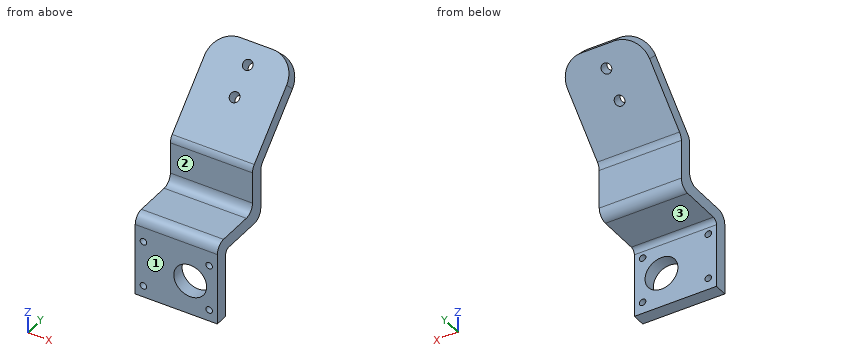
```python
from build123d import *

# Parameters (mm, degrees)
SKETCH1_W           = 50
SKETCH1_H           = 42
BOSS_EXTRUDE1_DEPTH = 8
SKETCH2_R           = 2
SKETCH2_R_2         = 10
CUT_EXTRUDE2_DEPTH  = 12
SKETCH6_W           = 50
SKETCH6_H           = 8
BOSS_EXTRUDE3_DEPTH = 33
SWEEP2_START        = -25
SWEEP2_DEPTH        = 50
FILLET1_R           = 6
FILLET2_R           = 3
SKETCH8_R           = 3
CUT_EXTRUDE3_DEPTH  = 38
FILLET3_R           = 15


# Read off the part's stored shape, not the designer's step: Sweep2
with BuildPart() as part:
    # Sketch1 → Boss-Extrude1 (new body)
    with BuildSketch(Plane(origin=(0, 0, 0), x_dir=(1, 0, 0), z_dir=(0, 1, 0))):
        Rectangle(SKETCH1_W, SKETCH1_H)
    extrude(amount=BOSS_EXTRUDE1_DEPTH)

    # Sketch2 → Cut-Extrude2 (cut)
    with BuildSketch(Plane(origin=(0, 8, 0), x_dir=(1, 0, 0), z_dir=(0, 1, 0))):
        with Locations(Location((-20, 14, 0), (0, 0, 270))):
            Circle(SKETCH2_R)
        with Locations(Location((20, 14, 0), (0, 0, 270))):
            Circle(SKETCH2_R)
        with Locations(Location((20, -14, 0), (0, 0, 270))):
            Circle(SKETCH2_R)
        with Locations(Location((-20, -14, 0), (0, 0, 270))):
            Circle(SKETCH2_R)
        with Locations(Location((8.5, 0, 0), (0, 0, 270))):
            Circle(SKETCH2_R_2)
    extrude(amount=-CUT_EXTRUDE2_DEPTH, mode=Mode.SUBTRACT)

    # Sketch6 → Boss-Extrude3 (add)
    with BuildSketch(Plane.XZ):
        with Locations((0, 25)):
            Rectangle(SKETCH6_W, SKETCH6_H)
    extrude(amount=-BOSS_EXTRUDE3_DEPTH)

    # Sweep2 outline → Sweep2 (add)
    with BuildSketch(Plane.YZ.offset(SWEEP2_START)):
        Polygon((33, 29), (33, 21), (42, 21), (42, 53.343145751), (83.254833996, 94.597979746), (77.597979746, 100.254833996), (34, 56.656854249), (34, 29), align=None)
    extrude(amount=SWEEP2_DEPTH)

    # Fillet1
    fillet1_edges = [part.edges().sort_by_distance(p)[0] for p in [
        (0, 0, 29),
        (0, 34, 56.656854249),
        (0, 42, 53.343145751),
        (0, 34, 29),
        (0, 42, 21),
    ]]
    fillet(fillet1_edges, radius=FILLET1_R)

    # Fillet2
    fillet2_edges = [part.edges().sort_by_distance(p)[0] for p in [
        (0, 8, 21),
    ]]
    fillet(fillet2_edges, radius=FILLET2_R)

    # Sketch8 → Cut-Extrude3 (cut)
    with BuildSketch(Plane(origin=(0, -11.328427125, 11.328427125), x_dir=(1, 0, 0), z_dir=(0, -0.7071067811865465, 0.7071067811865487))):
        with Locations(Location((0, 95.76093065, 0), (0, 0, 270))):
            Circle(SKETCH8_R)
        with Locations(Location((0, 113.76093065, 0), (0, 0, 270))):
            Circle(SKETCH8_R)
    extrude(amount=-CUT_EXTRUDE3_DEPTH, mode=Mode.SUBTRACT)

    # Fillet3
    fillet3_edges = [part.edges().sort_by_distance(p)[0] for p in [
        (-25, 80.426406871, 97.426406871),
        (25, 80.426406871, 97.426406871),
    ]]
    fillet(fillet3_edges, radius=FILLET3_R)


solid = part.part
```
Build history of the part. All positions in model axes, mm. Face numbers are marked on the shaded views. A direction names the side the tool comes from. Coordinates: 2 decimals unless noted, no trailing zeros. Write each loop counter-clockwise with the first axis right and the second up, starting at its lowest first coordinate (ties: lowest second). Pieces come first, ordered by that corner, then holes.
1. Drill centre lines: probe 1 along X at (y, z) = (5, -14); probe 2 along X at (y, z) = (2, 0); probe 3 along Z at (x, y) = (-14, 13). Where is each one in solid material? Low to high.
Answer block:
probe 1: x = -25 to -22, -18 to 18, 22 to 25
probe 2: x = -25 to -1.5, 18.5 to 25
probe 3: z = 21 to 29
2. Band-saw the part on B-B, the plane z = 0. Give the cut face in (x, y).
Answer block:
outline: (-25, 0) - (-1.5, 0) - (-1.5, 8) - (-25, 8) - close; (18.5, 0) - (25, 0) - (25, 8) - (18.5, 8) - close
3. Band-saw the part on C-C, the plane x = -20. Give the cut face in (y, z).
Answer block:
outline: (0, -21) - (8, -21) - (8, -16) - (0, -16) - close; (0, -12) - (8, -12) - (8, 12) - (0, 12) - close; (0, 16) - (8, 16) - (8, 18) arc R3 cw to (11, 21) - (36, 21) arc R6 ccw to (42, 27) - (42, 50.86) arc R6 cw to (43.76, 55.1) - (80.55, 91.9) - (74.9, 97.55) - (35.76, 58.41) arc R6 ccw to (34, 54.17) - (34, 35) arc R6 cw to (28, 29) - (6, 29) arc R6 ccw to (0, 23) - close
4. Band-saw the part on D-D, the plane x = 13.5. Give the cut face in (y, z), and give its area (3 significant figures).
Answer block:
outline: (0, -21) - (8, -21) - (8, -8.66) - (0, -8.66) - close; (0, 8.66) - (8, 8.66) - (8, 18) arc R3 cw to (11, 21) - (36, 21) arc R6 ccw to (42, 27) - (42, 50.86) arc R6 cw to (43.76, 55.1) - (82.96, 94.31) - (77.31, 99.96) - (35.76, 58.41) arc R6 ccw to (34, 54.17) - (34, 35) arc R6 cw to (28, 29) - (6, 29) arc R6 ccw to (0, 23) - close
area: 1,210 mm2
5. 3-axis set-ups, long thin cutter, end or side, ignore diameter. For the marked faces 1, 2 and 3: which of +Z, -Z, +X, -X, +Y, -Y reach the whole face in a straight line?
Answer block:
face 1: +Z, -Z, +X, -X, -Y
face 2: +Z, +X, -X, -Y
face 3: -Z, +X, -X, +Y
6. Band-saw the part on A-A, the plane z = -14. Give the cut face in (x, y), and give its area (3 significant figures).
Answer block:
outline: (-25, 0) - (-22, 0) - (-22, 8) - (-25, 8) - close; (-18, 0) - (18, 0) - (18, 8) - (-18, 8) - close; (22, 0) - (25, 0) - (25, 8) - (22, 8) - close
area: 336 mm2
7. Drop flat-ended pins along their axis: pin 1 (15.5 mm diameter, centred on x = -10.5, z = 48, fed in from -Y); pin 2 (4 mm diameter, centred on x = 7.5, y = 30, fed in from +Z); pin 3 (12.5 mm diameter, centred on x = 7.5, y = 20.5, fed in from -Z); pin 4 (12 mm diameter, centred on y = 29.5, z = 57, fed in from -X). Give the stop position or say it passes through.
Answer block:
pin 1: stops at y = 34
pin 2: stops at z = 30.53
pin 3: stops at z = 21
pin 4: stops at x = -25
